Here's the drawing with two shaded views (mm, measured from the low corner). I have some questions. A direction names the side the tool comes from. Give positions to 0.01 mm unless a question says otherwise; leave off trailing zeros. Order: outer loops, then holes, each group sorted by start corner. A loop starts at its lowest first (then second) coordinate and runs counter-clockwise, first axis right, second up. Notation, with made-up numbers: M 70.25,56.25 L 86.25,56.25 A13 cw 86.25,81.25 Z; hole C 27,45.25 d5. An arc over 180 degrees is marked long. Use a Markdown table: item, result. Add a question column.
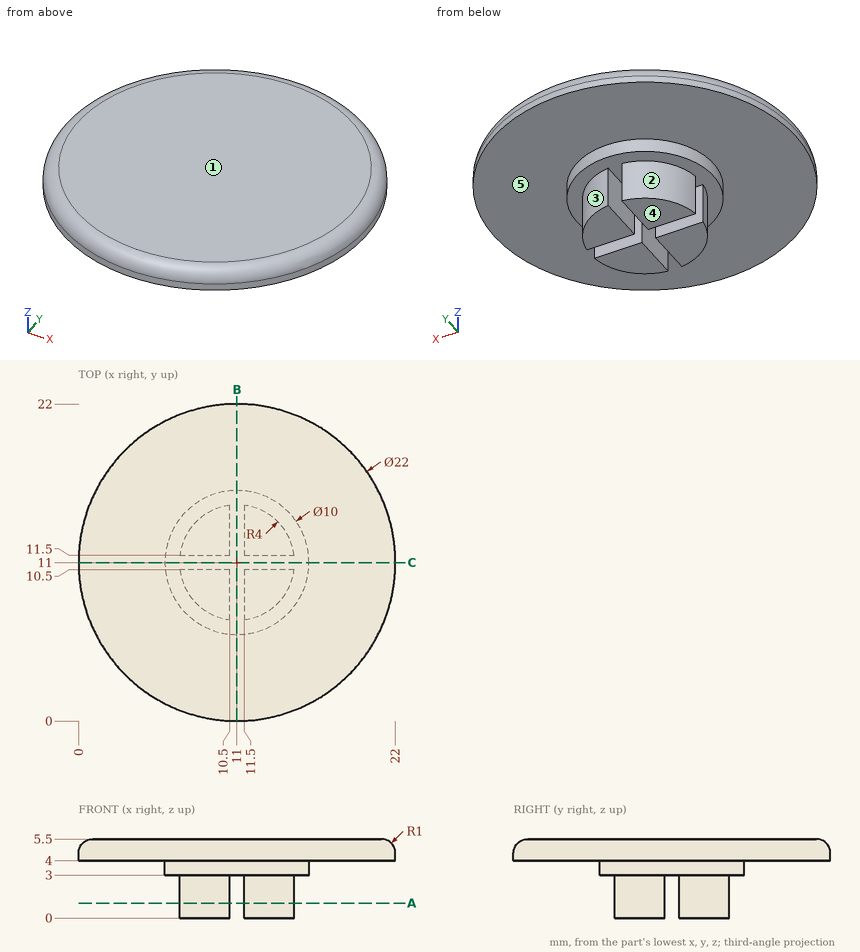
1) Please list where these lines run through material, in increasing order: line 1 (Z direction, x = 10.75, y = 4); line 2 (X direction, y = 12, z = 2.8); line 3 (Y direction, x = 10.25, z = 2.95). Write a range as from..to.
2) For pin 1 (0.9 mm diameter, centred on y = 8, z = 1.5, fed in from -X); pin 2 (0.9 mm diameter, centred on x = 8, z = 2, fed in from -Y); pin 3 (3 mm diameter, centred on y = 15.5, z = 3, fed in from +X), each with a flat end and sliding along its axis, tell me the tip position at first contact or that it passes through.
3) For the marked faces 1, 2, 3, 4 and 5, which set-ups out of +Z, -Z, +X, -X, +Y, -Y let a thin tool reach every point of the face, with its end or its side?
4) Suppose I cut it at B-B on x = 11. Please give me the cut outline in (y, z).
5) Suppose I cut it at A-A on z = 1.05. Please give me the cut outline in (x, y).
Values found:
| question | item | result |
|---|---|---|
| 1 | line 1 | z = 4..5.5 |
| 1 | line 2 | x = 7.13..10.5, 11.5..14.87 |
| 1 | line 3 | y = 7.07..10.5, 11.5..14.93 |
| 2 | pin 1 | stops at x = 7.92 |
| 2 | pin 2 | stops at y = 7.92 |
| 2 | pin 3 | stops at x = 21.47 |
| 3 | face 1 | +Z, +X, -X, +Y, -Y |
| 3 | face 2 | -Z, -X, +Y |
| 3 | face 3 | -Z, +X, +Y |
| 3 | face 4 | -Z, +X, -X, +Y, -Y |
| 3 | face 5 | -Z |
| 4 | outline | M 0,4 L 6,4 L 6,3 L 16,3 L 16,4 L 22,4 L 22,4.5 A1 ccw 21,5.5 L 1,5.5 A1 ccw 0,4.5 Z |
| 5 | outline | M 7.03,10.5 A4 ccw 10.5,7.03 L 10.5,10.5 Z; M 7.03,11.5 L 10.5,11.5 L 10.5,14.97 A4 ccw Z; M 11.5,7.03 A4 ccw 14.97,10.5 L 11.5,10.5 Z; M 11.5,11.5 L 14.97,11.5 A4 ccw 11.5,14.97 Z |
